Autodesk Fusion 360 part; units mm, degrees
sketch "Sketch1" plane through (0, 0, 0) normal (1, 0, 0) x (0, 1, 0)
  line L0 (-12.5, 0) -> (12.5, 0)
  line L1 (12.5, 0) -> (12.5, 25)
  line L2 (12.5, 25) -> (9.5, 25)
  line L3 (9.5, 25) -> (9.5, 3)
  line L4 (9.5, 3) -> (-12.5, 3)
  line L5 (-12.5, 3) -> (-12.5, 0)
  dimension "d2" = 25
  dimension "d3" = 25
  dimension "d4" = 3
  dimension "d5" = 22
  dimension "d6" = 22
extrude "Extrude1" add sketch "Sketch1" along normal mid plane 1500
sketch "Sketch2" plane through (0, 0, 0) normal (0, 0, -1) x (1, 0, 0)
  line L0 (-750, -12.5) -> (750, -12.5)
  line L1 (750, -12.5) -> (750, 12.5)
  line L2 (750, 12.5) -> (-750, 12.5)
  line L3 (-750, 12.5) -> (-750, -12.5)
  line L4 (-750, 0) -> (-730, 0) construction
  line L5 (-730, 0) -> (-660, 0) construction
  line L6 (750, 0) -> (730, 0) construction
  line L7 (730, 0) -> (660, 0) construction
  dimension "d9" = 20
  dimension "d10" = 70
  dimension "d11" = 20
  dimension "d12" = 70
hole "Hole1" at (-660, 0, 0) at (-730, 0, 0) at (730, 0, 0) at (660, 0, 0) direction (0, 0, 1) diameter 5.5 depth 3 tip angle 180
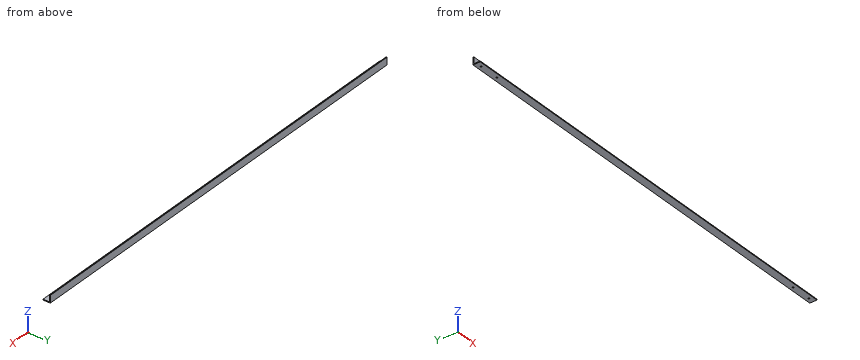
Part model, mm, in its own coordinate system. Round coordinates to 2 decimals unless told otherwise and drop trailing zeros. Loops run counter-clockwise (first coordinate to the right, second up) from the corner with the lowest first, then second, coordinate; pieces in that order, holes last.
1. Flat gauge pins, fed straight in: pin 1 (12 mm diameter, centred on x = 66, y = -6, fed in from +Z); pin 2 (4.5 mm diameter, centred on x = 730, y = 0, fed in from +Z); pin 3 (12 mm diameter, centred on x = 276, z = 10.5, fed in from -Y); pin 4 (12 mm diameter, centred on y = -5.5, z = 8, fed in from -X). Where does each tip first touch, or does it go through?
Solutions:
pin 1: stops at z = 3
pin 2: passes through
pin 3: stops at y = 9.5
pin 4: stops at x = -750
2. Slice it at B-B (z = 21). Give the cut face in (x, y).
Solutions:
outline: (-750, 9.5) - (750, 9.5) - (750, 12.5) - (-750, 12.5) - close
3. Drill centre lines: line 1 along X through (y, z) = (0, 1.55); line 2 along Y through (x, z) = (660, 1.35); line 3 along Z through (x, y) = (395, 7). Where is each one in solid material? Low to high.
Solutions:
line 1: x = -750 to -732.75, -727.25 to -662.75, -657.25 to 657.25, 662.75 to 727.25, 732.75 to 750
line 2: y = -12.5 to -2.75, 2.75 to 12.5
line 3: z = 0 to 3
4. Slice it at A-A (x = -350). Give the cut face in (y, z), and give its area (3 significant figures).
Solutions:
outline: (-12.5, 0) - (12.5, 0) - (12.5, 25) - (9.5, 25) - (9.5, 3) - (-12.5, 3) - close
area: 141 mm2
